```python
from build123d import *

# Parameters (mm, degrees)
CROQUIS1_W              = 30
CROQUIS1_H              = 30
CROQUIS1_R              = 5.43144852
SALIENTE_EXTRUIR1_DEPTH = 3


with BuildPart() as part:
    # Croquis1 → Saliente-Extruir1 (new body)
    with BuildSketch(Plane.XY):
        Rectangle(CROQUIS1_W, CROQUIS1_H)
        with Locations((5.43144852, -5.43144852)):
            Circle(CROQUIS1_R, mode=Mode.SUBTRACT)
        with BuildLine():
            Line((-11, -11), (-11, -6.30958424))
            ThreePointArc((-11, -6.30958424), (-10.604257207, -6.798593887), (-10.043478261, -6.51351536))
            ThreePointArc((-10.043478261, -6.51351536), (-7.184032198, -2.669953099), (-2.962030371, -0.40630489))
            ThreePointArc((-2.962030371, -0.40630489), (-1.479948679, 0.371768463), (-0.44603831, 1.688200624))
            add(Edge.make_bspline(
                [(-0.44603831, 1.688200624), (0.600161472, 2.997780482), (1.259535405, 5.412607882), (3.723491408, 7.268772296), (6.075005948, 7.554534112), (8.017011232, 8.499729242), (7.239010254, 10.03791357)],
                knots=[0, 0, 0, 0, 0.408369394, 0.584001697, 0.707826515, 1, 1, 1, 1], degree=3))
            ThreePointArc((7.239010254, 10.03791357), (7.538453023, 10.597357036), (7.048023, 11))
            Line((7.048023, 11), (11, 11))
            Line((11, 11), (11, 4.715933429))
            ThreePointArc((11, 4.715933429), (10.551626523, 5.213260989), (10.010661191, 4.8186346))
            ThreePointArc((10.010661191, 4.8186346), (9.813510438, 4.116058971), (9.524664361, 3.445947877))
            add(Edge.make_bspline(
                [(4.653277623, 2.773397026), (6.138085687, 2.096565381), (8.467088589, 1.756469214), (9.524664361, 3.445947877)],
                knots=[0, 0, 0, 0, 1, 1, 1, 1], degree=3))
            add(Edge.make_bspline(
                [(-0.124019497, -1.647133295), (0.48560807, 0.564599921), (2.28878007, 2.613788972), (4.653277623, 2.773397026)],
                knots=[0.123819996, 0.123819996, 0.123819996, 0.123819996, 1, 1, 1, 1], degree=3))
            ThreePointArc((-0.124019497, -1.647133295), (-0.206307312, -2.120424053), (-0.309181236, -2.589670665))
            ThreePointArc((-0.309181236, -2.589670665), (-2.545566455, -7.037226259), (-6.51351536, -10.043478261))
            ThreePointArc((-6.51351536, -10.043478261), (-6.798593887, -10.604257207), (-6.30958424, -11))
            Line((-6.30958424, -11), (-11, -11))
        make_face(mode=Mode.SUBTRACT)
        with Locations((-5.43144852, 5.43144852)):
            Circle(CROQUIS1_R, mode=Mode.SUBTRACT)
    extrude(amount=SALIENTE_EXTRUIR1_DEPTH)


solid = part.part
```
Here's how the part is built. I have some questions about the finished solid (model axes, mm). A direction names the side the tool comes from. Give positions to 0.01 mm unless a question says otherwise; leave off trailing zeros. Loops run counter-clockwise (first coordinate to the right, second up) from the corner with the lowest first, then second, coordinate; pieces in that order, holes last. Notation, with made-up numbers: M 34,0.5 L 60,0.5 A19 cw 60,22.5 Z; hole C 26,-1.75 d9. An arc over 180 degrees is marked long. Use one line per item in the form item = value. Start each with the question number.
Q1. If we section it at A-A (y = -9): Write out the boundary of the cut face in (x, z).
Q2. Which directions (+Z, -Z, +X, -X, +Y, -Y) give clear straight access to the entire face, cutting with the end or side of a thin tool? Please do faces 1 (the cylindrical face through (9.82, 4.13, 1.48)), 2 (the flat face through (-15, 0, 1)).
Q3. If we section it at B-B (x = -8.5): Write out the boundary of the cut face in (y, z), then the cut area to 3 significant figures.
Q4. Will this pin go through, and if not, where does the flat tip stop? pin 1 Ø6.5 at (x, y) = (-5.43, 5.43) entering from -Z.
Q5. If we section it at C-C (z = 1.15): State how many separate pieces and enclosed holes the cut face has, then the cut area to 3 significant figures.
Q6. Thinking about a two-plate mould opening in Y: for faces 3 (the flat face through (0, 15, 1)), 4 (the flat face through (3, 0, 3)), 5 (the flat face through (-9, -11, 1)), which applies, +Y half, -Y half, draft (parallel to the pull), parting line (faces both ways), or undercut?
Q7. I need wall thicknesses on line 1 along Y through (x, z) = (6.5, 1.95); line 2 along Y through (x, z) = (-7.5, 0.4); line 3 along X through (y, z) = (1.5, 1.6). Which ranges of each line are inside material? Lowest first, please.
Taken from the geometry:
q1.outline = M -15,0 L -11,0 L -11,3 L -15,3 Z; M -4.68,0 L 1.34,0 L 1.34,3 L -4.68,3 Z; M 9.53,0 L 15,0 L 15,3 L 9.53,3 Z
q2.face_1 = +Z, -Z
q2.face_2 = +Z, -Z, -X, +Y, -Y
q3.outline = M -15,0 L -11,0 L -11,3 L -15,3 Z; M -4.02,0 L 0.95,0 L 0.95,3 L -4.02,3 Z; M 9.91,0 L 15,0 L 15,3 L 9.91,3 Z
q3.area = 42.2 mm^2
q4.pin_1 = through
q5.separate_pieces = 1
q5.enclosed_holes = 3
q5.area = 580 mm^2
q6.face_3 = +Y half
q6.face_4 = draft
q6.face_5 = undercut
q7.line_1 = -15 to -10.76, -0.11 to 2.25, 7.92 to 15
q7.line_2 = -15 to -11, -2.95 to 0.41, 10.45 to 15
q7.line_3 = -15 to -9.18, -1.68 to -0.54, 1.78 to 15
